Source: CAD feature listing. Evaluate the final solid. Frame: model axes, mm. A direction names the side the tool comes from. Round coordinates to 2 decimals unless told otherwise and drop trailing zeros. Order: outer loops, then holes, each group sorted by start corner. A loop starts at its lowest first (then second) coordinate and runs counter-clockwise, first axis right, second up. Notation, with made-up numbers: (78, 84) - (130, 84) arc R12 cw to (130, 97) - close; hole circle Ø2 at (63, 47). An arc over 180 degrees is marked (long way). Return JSON: item names as keys, results as strings. Group by question number.
1) Mould query, pull axis Z, two halves, no side actions, for faces 1 (the flat face through (-45, 9.9, -1.6)), 2 (the flat face through (54.062, 16.807, -11.458)), 3 (the cylindrical face through (54, 10, -2)). Classes: pulls with the +Z half, pulls with the -Z half, needs draft (parallel to the pull), parting line crosses it, or undercut.
2) Ray query, line 1 (Z direction, x = 62.25, y = 10); line 2 (X direction, y = 13, z = -11); line 3 (X direction, y = 8.75, z = -6). Return the intervals inside material, ascending. Write a range as from..to.
3) Section A-A, the plane z = -8.5. Return loops of the section in (x, y) (3 decimals).
4) Section C-C, the plane x = -24.5. Return loops of the section in (y, z).
5) Section D-D, the plane y = 10. Give the number of separate pieces and of enclosed holes in the cut face, plus the area to 3 significant figures.
6) Contact query for flat-ended pins moving along their axis: P1, Ø8, axis at y = 14.5, z = 2, coming from the -X side; P2, Ø6.5, axis at y = 10, z = -6.5, coming from the -X side; P3, Ø0.9, axis at y = 12.5, z = -1.5, coming from the +X side; P4, Ø4, axis at x = -69, y = 9.5, coming from the -Z side. Output: stop coordinate, or through.
7) Section B-B, the plane z = 2.5. Return loops of the section in (x, y) (3 decimals).
8) Access query for faces 4 (the flat face through (-60, 10.1, -11.3)), 5 (the flat face through (69, 12.5, 10)), 6 (the flat face through (45, 9.9, -1.6)). Directions: +Z, -Z, +X, -X, +Y, -Y. A direction counts if a zero-diameter tool reaches every point of the face in a straight line with its end or side. Return the directions, or none.
```python
from build123d import *

# Parameters (mm, degrees)
BOSS_EXTRUDE1_DEPTH = 20
SKETCH3_W           = 17
SKETCH3_H           = 20
SKETCH2_W           = 17
SKETCH2_H           = 20.004497681
SKETCH5_W           = 5
SKETCH5_H           = 5
BOSS_EXTRUDE2_DEPTH = 20
SKETCH6_R           = 2.55
CUT_EXTRUDE1_DEPTH  = 12.47988838
SKETCH8_W           = 17
SKETCH8_H           = 20
SKETCH7_W           = 3
SKETCH7_H           = 20
SKETCH9_R           = 6.5
CUT_EXTRUDE2_DEPTH  = 30


with BuildPart() as part:
    # Sketch1 → Boss-Extrude1 (new body)
    with BuildSketch(Plane.XY):
        Polygon((-66.745, 0), (66.745, 0), (66.320821408, 20), (-66.320821408, 20), align=None)
    extrude(amount=BOSS_EXTRUDE1_DEPTH)

    # Sketch3 → Loft1 section 0
    with BuildSketch(Plane(origin=(60, 0, 0), x_dir=(0, 0, -1), z_dir=(1, 0, 0))):
        with Locations((8.5, 10)):
            Rectangle(SKETCH3_W, SKETCH3_H)
    # Sketch2 → Loft1 section 1
    with BuildSketch(Plane(origin=(66.71499035, 1.414953534, 0), x_dir=(0, 0, -1), z_dir=(0.999775167, 0.021204161, 0))):
        with Locations((8.5, 8.586977106)):
            Rectangle(SKETCH2_W, SKETCH2_H)
    loft1 = loft()

    # Sketch5 → Boss-Extrude2 (add)
    with BuildSketch(Plane.XY.offset(20)):
        with Locations((68.97988838, 10)):
            Rectangle(SKETCH5_W, SKETCH5_H)
    boss_extrude2 = extrude(amount=-BOSS_EXTRUDE2_DEPTH)

    # Mirror2: Boss-Extrude2 across plane
    add(boss_extrude2.mirror(Plane(origin=(0, 0, 0), x_dir=(0, 0, 1), z_dir=(1, 0, 0))))

    # Sketch6 → Cut-Extrude1 (cut, through all)
    with BuildSketch(Plane.ZY.offset(-60)):
        with Locations((-8.5, 10)):
            Circle(SKETCH6_R)
    cut_extrude1 = extrude(amount=-CUT_EXTRUDE1_DEPTH, mode=Mode.SUBTRACT)

    # Sketch8 → Loft2 section 0
    with BuildSketch(Plane.ZY.offset(-60)):
        with Locations((-8.5, 10)):
            Rectangle(SKETCH8_W, SKETCH8_H)
    # Sketch7 → Loft2 section 1
    with BuildSketch(Plane(origin=(45, 0, 0), x_dir=(0, 0, -1), z_dir=(1, 0, 0))):
        with Locations((1.5, 10)):
            Rectangle(SKETCH7_W, SKETCH7_H)
    loft2 = loft()

    # Sketch9 → Cut-Extrude2 (cut)
    with BuildSketch(Plane(origin=(60, 0, 0), x_dir=(0, 0, -1), z_dir=(1, 0, 0))):
        with Locations((8.5, 10)):
            Circle(SKETCH9_R)
    cut_extrude2 = extrude(amount=-CUT_EXTRUDE2_DEPTH, mode=Mode.SUBTRACT)

    # Mirror3: Loft1, Cut-Extrude1, Loft2, Cut-Extrude2 across plane
    add(loft1.mirror(Plane(origin=(0, 0, 0), x_dir=(0, 0, 1), z_dir=(1, 0, 0))))
    add(cut_extrude1.mirror(Plane(origin=(0, 0, 0), x_dir=(0, 0, 1), z_dir=(1, 0, 0))), mode=Mode.SUBTRACT)
    add(loft2.mirror(Plane(origin=(0, 0, 0), x_dir=(0, 0, 1), z_dir=(1, 0, 0))))
    add(cut_extrude2.mirror(Plane(origin=(0, 0, 0), x_dir=(0, 0, 1), z_dir=(1, 0, 0))), mode=Mode.SUBTRACT)


solid = part.part
```
Geometry check:
{
 "1": {"face 1": "needs draft", "face 2": "pulls with the -Z half", "face 3": "undercut"},
 "2": {"line 1": "-17..-11.05, -5.95..20", "line 2": "-66.47..-60, 60..66.47", "line 3": "-66.56..-60, 60..66.56"},
 "3": {"outline": "(-66.745, 0) - (-50.893, 0) - (-50.893, 3.5) - (-60, 3.5) - (-60, 7.45) - (-66.587, 7.45) - close; (-66.479, 12.55) - (-60, 12.55) - (-60, 16.5) - (-50.893, 16.5) - (-50.893, 20) - (-66.321, 20) - close; (50.893, 0) - (66.745, 0) - (66.587, 7.45) - (60, 7.45) - (60, 3.5) - (50.893, 3.5) - close; (50.893, 16.5) - (60, 16.5) - (60, 12.55) - (66.479, 12.55) - (66.321, 20) - (50.893, 20) - close"},
 "4": {"outline": "(0, 0) - (20, 0) - (20, 20) - (0, 20) - close"},
 "5": {"separate pieces": "3", "enclosed holes": "0", "area": "3,080 mm2"},
 "6": {"P1": "x = -71.48", "P2": "x = -66.6", "P3": "x = 66.49", "P4": "z = 0"},
 "7": {"outline": "(-71.48, 7.5) - (-66.586, 7.5) - (-66.745, 0) - (66.745, 0) - (66.586, 7.5) - (71.48, 7.5) - (71.48, 12.5) - (66.48, 12.5) - (66.321, 20) - (-66.321, 20) - (-66.48, 12.5) - (-71.48, 12.5) - close"},
 "8": {"face 4": "none", "face 5": "+Z, -Z, +X, +Y", "face 6": "-Z, +Y, -Y"}
}
